Autodesk Inventor part; units mm, degrees
ref_plane "Work Plane1" through (-43.4917, 1.5875, -7.62) normal (0, -1, 0) x (1, 0, 0)
ref_plane "YZ Plane" through (0, 0, 0) normal (1, 0, 0) x (0, 1, 0)
ref_plane "XZ Plane" through (0, 0, 0) normal (0, 1, 0) x (-1, 0, 0)
ref_plane "Work Plane1" through (-43.4917, 1.5875, -7.62) normal (0, -1, 0) x (1, 0, 0)
sketch "Sketch3" plane through (-43.4917, 1.5875, -7.62) normal (0, -1, 0) x (1, 0, 0)
  line L0 (-106.9189, -23.7145) -> (70.8811, -23.7145)
  line L1 (70.8811, -23.7145) -> (70.8811, 65.1855)
  line L2 (70.8811, 65.1855) -> (-106.9189, 65.1855)
  line L3 (-106.9189, 65.1855) -> (-106.9189, -23.7145)
  line L4 (-106.9189, -23.7145) -> (70.8811, -23.7145)
  line L5 (70.8811, -23.7145) -> (70.8811, -18.6345)
  line L6 (70.8811, -18.6345) -> (-106.9189, -18.6345)
  line L7 (-106.9189, -18.6345) -> (-106.9189, -23.7145)
  line L8 (-106.9189, 65.1855) -> (-101.8389, 65.1855)
  line L9 (-101.8389, 65.1855) -> (-101.8389, -23.7145)
  line L10 (-101.8389, -23.7145) -> (-106.9189, -23.7145)
  line L11 (-106.9189, -23.7145) -> (-106.9189, 65.1855)
  line L12 (-106.9189, 65.1855) -> (70.8811, 65.1855)
  line L13 (70.8811, 65.1855) -> (70.8811, 60.1055)
  line L14 (70.8811, 60.1055) -> (-106.9189, 60.1055)
  line L15 (-106.9189, 60.1055) -> (-106.9189, 65.1855)
  line L16 (70.8811, -23.7145) -> (65.8011, -23.7145)
  line L17 (65.8011, -23.7145) -> (65.8011, 65.1855)
  line L18 (65.8011, 65.1855) -> (70.8811, 65.1855)
  line L19 (70.8811, 65.1855) -> (70.8811, -23.7145)
  point P0 (43.4917, 7.62)
  dimension "d1" = 177.8
  dimension "d2" = 88.9
  dimension "d3" = 5.08
  dimension "d4" = 5.08
  dimension "d5" = 5.08
  dimension "d6" = 5.08
extrude "Extrusion1" add sketch "Sketch3" against normal blind 76.2 contours L3 L2 L9 L14 | L9 L2 L17 L14 | L17 L2 L1 L14
extrude "Extrusion2" cut sketch "Sketch3" against normal blind 76.2 contours L3 L6 L9 L0 | L3 L14 L9 L6 | L3 L2 L9 L14
extrude "Extrusion3" cut sketch "Sketch3" against normal blind 76.2 contours L3 L6 L9 L0 | L9 L6 L17 L0 | L3 L14 L9 L6 | L17 L6 L1 L0 | L3 L2 L9 L14 | L17 L14 L1 L6 | L17 L2 L1 L14
extrude "Extrusion4" add sketch "Sketch3" against normal blind 76.2 contours L3 L6 L9 L0 | L3 L14 L9 L6 | L3 L2 L9 L14
extrude "Extrusion5" add sketch "Sketch3" against normal blind 76.2 contours L17 L6 L1 L0 | L17 L14 L1 L6 | L17 L2 L1 L14
extrude "Extrusion6" add sketch "Sketch3" against normal blind 76.2 contours L3 L6 L9 L0 | L9 L6 L17 L0 | L17 L6 L1 L0
extrude "Extrusion7" add sketch "Sketch3" along normal blind 5.08 contours L9 L14 L17 L6
extrude "Extrusion8" add sketch "Sketch3" along normal blind 5.08 contours L17 L6 L1 L0 | L17 L14 L1 L6 | L17 L2 L1 L14
extrude "Extrusion9" add sketch "Sketch3" along normal blind 5.08 contours L3 L6 L9 L0 | L9 L6 L17 L0 | L17 L6 L1 L0
extrude "Extrusion10" add sketch "Sketch3" along normal blind 5.08 contours L3 L6 L9 L0 | L3 L14 L9 L6 | L3 L2 L9 L14
extrude "Extrusion11" add sketch "Sketch3" along normal blind 5.08 contours L3 L2 L9 L14 | L9 L2 L17 L14 | L17 L2 L1 L14
properties part number "enclosure"
Check sheet for the modelled part. Datum: model origin and axes. Units: mm. A direction names the side the tool comes from. Round coordinates to 2 decimals unless told otherwise and drop trailing zeros. Loops run counter-clockwise (first coordinate to the right, second up) from the corner with the lowest first, then second, coordinate; pieces in that order, holes last. Notation, with made-up numbers: M 68.5,-27.75 L 72.5,-27.75 A9 cw 72.5,-21.75 Z; hole C 13,66 d3. An arc over 180 degrees is marked long. One line per item, written item: value.
(1) Release check for a two-part mould opening along X. For faces 1 (the face through (-150.411, 37, 14)), 2 (the face through (-63, 1.588, 14)), 3 (the face through (-60, 39, 52.486)), 4 (the face through (-63, -3.492, 14)) record: +X half, -X half, draft (parallel to the pull), parting line (faces both ways), or undercut.
Computed values:
face 1: -X half
face 2: undercut
face 3: undercut
face 4: draft
(2) Access from +Z, -Z, +X, -X, +Y, -Y to the whole of each face (thin tool, end or side, straight path). Record for faces 5 (the face through (-63, 37, -31.334)), 6 (the face through (-60, 39, -26.254)).
Computed values:
face 5: -Z, +X, -X, +Y, -Y
face 6: +Y
(3) Sectioned sample at A-A, the plane y = 38. Record the cut outline in (x, z).
Computed values:
outline: M -150.41,-31.33 L 27.39,-31.33 L 27.39,57.57 L -150.41,57.57 Z; hole M -145.33,-26.25 L 22.31,-26.25 L 22.31,52.49 L -145.33,52.49 Z
(4) Thickness scan on line 1 (Z direction, x = -20, y = 40.5); line 2 (X direction, y = 15.5, z = 47); line 3 (Y direction, x = 5, z = -22). Record the ranges inside material, lowest first.
Computed values:
line 1: z = -31.33 to -26.25, 52.49 to 57.57
line 2: x = -150.41 to -145.33, 22.31 to 27.39
line 3: y = -3.49 to 1.59
(5) Sectioned sample at B-B, the plane x = -36. Record the cut outline in (y, z).
Computed values:
outline: M -3.49,-31.33 L 77.79,-31.33 L 77.79,-26.25 L 1.59,-26.25 L 1.59,52.49 L 77.79,52.49 L 77.79,57.57 L -3.49,57.57 Z
(6) Sectioned sample at C-C, the plane z = 36.5. Record the cut outline in (x, y).
Computed values:
outline: M -150.41,-3.49 L 27.39,-3.49 L 27.39,77.79 L 22.31,77.79 L 22.31,1.59 L -145.33,1.59 L -145.33,77.79 L -150.41,77.79 Z
(7) Depth check by flat-ended pin: pin 1 Ø1.5 at (x, z) = (-97, 26) entering from +Y. Enter the tip coordinate at first touch or a pass-through.
Computed values:
pin 1: stops at y = 1.59
